Autodesk Inventor part; units mm, degrees
ref_plane "Work Plane1" through (0, 0, -15) normal (0, 0, 1) x (1, 0, 0)
ref_plane "YZ Plane" through (0, 0, 0) normal (1, 0, 0) x (0, 1, 0)
ref_plane "XZ Plane" through (0, 0, 0) normal (0, 1, 0) x (-1, 0, 0)
sketch "Sketch1" plane through (0, 0, 0) normal (0, 0, 1) x (1, 0, 0)
  line L0 (0, 0) -> (25, 0)
  line L1 (25, 0) -> (25, 40)
  line L2 (25, 40) -> (0, 40)
  line L3 (0, 40) -> (0, 0)
  dimension "d1" = 25
  dimension "d2" = 40
  dimension "d3" = 25
extrude "Extrusion1" add sketch "Sketch1" against normal blind 30
sketch "Sketch2" plane through (25, 0, 0) normal (1, 0, 0) x (0, 0, -1)
  line L0 (0, 0) -> (30, 0)
  circle A0 centre (15, 6.56) radius 2.46
extrude "Extrusion2" cut sketch "Sketch2" against normal blind 30
sketch "Sketch3" plane through (0, 0, 0) normal (-1, 0, 0) x (0, 0, 1)
  line L0 (0, 0) -> (-30, 0)
  line L1 (-25.05, 0) -> (-4.95, 0)
  line L2 (-4.95, 0) -> (-4.95, 33.12)
  line L3 (-4.95, 33.12) -> (-25.05, 33.12)
  line L4 (-25.05, 33.12) -> (-25.05, 0)
  dimension "d11" = 20.1
extrude "Extrusion3" cut sketch "Sketch3" against normal blind 20
sketch "Sketch4" plane through (0, 0, 0) normal (0, -1, 0) x (1, 0, 0)
  line L0 (20, -4.95) -> (20, -25.05)
  line L1 (20, -15) -> (25, -15)
  line L2 (25, 0) -> (25, -30)
  line L3 (20, -8.025) -> (25, -8.025)
  line L4 (25, -8.025) -> (25, -21.975)
  line L5 (25, -21.975) -> (20, -21.975)
  line L6 (20, -21.975) -> (20, -8.025)
  line L7 (20, -8.025) -> (25, -21.975) construction
  line L8 (25, -8.025) -> (20, -21.975) construction
  line L9 (25, -12.54) -> (25, -17.46)
  point P0 (0, 0)
  point P1 (22.5, -15)
  dimension "d14" = 13.95
extrude "Extrusion4" add sketch "Sketch4" along normal blind 15
sketch "Sketch5" plane through (20, 0, 0) normal (-1, 0, 0) x (0, 0, 1)
  circle A0 centre (-15, 6.56) radius 2.46
  circle A1 centre (-15, 6.56) radius 4.7025
  circle A2 centre (-15, 6.56) radius 2.46
  circle A3 centre (-15, 6.56) radius 2.46
  point P0 (0, 0)
  dimension "d17" = 9.405
extrude "Extrusion5" cut sketch "Sketch5" against normal blind 2.1
sketch "Sketch6" plane through (25, 0, 0) normal (1, 0, 0) x (0, 0, -1)
  circle A0 centre (15, 6.56) radius 4.7025
  line L0 (15, 6.56) -> (15, 23.56)
  circle A1 centre (15, 23.56) radius 2.46
  point P0 (0, 0)
  dimension "d20" = 17
  dimension "d21" = 4.92
extrude "Extrusion6" cut sketch "Sketch6" against normal blind 10 contours A1
sketch "Sketch7" plane through (20, 0, 0) normal (-1, 0, 0) x (0, 0, 1)
  circle A0 centre (-15, 23.56) radius 2.46
  circle A1 centre (-15, 23.56) radius 4.7025
  point P0 (0, 0)
  dimension "d24" = 9.405
extrude "Extrusion7" cut sketch "Sketch7" against normal blind 2.1
sketch "Sketch9" plane through (25, 0, 0) normal (1, 0, 0) x (0, 0, -1)
  circle A0 centre (15, 6.56) radius 2.46
  circle A1 centre (15, 6.56) radius 2.46
  circle A2 centre (15, 23.56) radius 2.46
  circle A3 centre (15, 23.56) radius 2.46
  line L0 (30, 40) -> (30, 0)
  line L1 (30, 0) -> (30, 40)
  line L2 (30, 40) -> (0, 40)
  line L3 (0, 40) -> (0, 0)
  line L4 (0, 0) -> (8.025, 0)
  line L5 (21.975, 0) -> (21.975, -15)
  line L6 (21.975, -15) -> (8.025, -15)
  line L7 (8.025, -15) -> (8.025, 0)
  line L8 (0, 0) -> (8.025, 0)
  line L9 (21.975, 0) -> (30, 0)
extrude "Extrusion8" add sketch "Sketch9" along normal blind 5
sketch "Sketch10" plane through (0, 40, 0) normal (0, 1, 0) x (1, 0, 0)
  line L0 (0, 30) -> (30, 30)
  line L1 (30, 0) -> (0, 0)
  line L2 (0, 30) -> (30, 30)
  line L3 (30, 30) -> (30, 0)
  line L4 (30, 0) -> (0, 0)
  line L5 (0, 0) -> (0, 30)
extrude "Extrusion9" add sketch "Sketch10" along normal blind 30
sketch "Sketch12" plane through (30, 0, 0) normal (1, 0, 0) x (0, 0, -1)
  circle A0 centre (15, 6.56) radius 2.46
  line L0 (15, 6.56) -> (15, 15.06)
  circle A1 centre (15, 15.06) radius 2.525
  point P0 (0, 0)
  dimension "d31" = 8.5
  dimension "d33" = 5.05
extrude "Extrusion10" cut sketch "Sketch12" against normal blind 30 contours A1
sketch "Sketch14" plane through (0, 0, 0) normal (0, 0, 1) x (1, 0, 0)
  line L0 (30, 70) -> (0, 70)
  line L1 (0, 70) -> (0, 85)
  line L2 (30, 100) -> (15, 115)
  line L3 (-12, 115) -> (15, 115)
  line L4 (30, 0) -> (30, 70)
  line L5 (30, 100) -> (30, 70)
  line L6 (-9.5, 113.5) -> (-12, 115)
  line L7 (-9.5, 101.5) -> (-12, 100)
  line L8 (-7, 107.5) -> (-9.5, 101.5)
  line L9 (-7, 107.5) -> (-9.5, 113.5)
  line L10 (0, 100) -> (0, 85)
  line L11 (0, 100) -> (-12, 100)
  point P0 (0, 0)
  dimension "d49" = 15
  dimension "d61" = 12
extrude "Extrusion12" add sketch "Sketch14" against normal blind 30
sketch "Sketch15" plane through (0, 0, -25.05) normal (-1, 0, 0) x (0, 0, 1)
  line L0 (0, 33.12) -> (20.1, 33.12)
  line L1 (20.1, 33.12) -> (20.1, 0)
  line L2 (0, 33.12) -> (20.1, 33.12)
  line L3 (20.1, 33.12) -> (20.1, 31.1)
  line L4 (20.1, 31.1) -> (0, 31.1)
  line L5 (0, 31.1) -> (0, 33.12)
  point P0 (25.05, 0)
  dimension "d57" = 2.02
extrude "Extrusion13" add sketch "Sketch15" against normal blind 20
sketch "Sketch19" plane through (0, 0, 0) normal (0, 0, 1) x (1, 0, 0)
  line L0 (0, 100) -> (0, 0)
  line L1 (0, 100) -> (-12, 100)
  line L2 (0, 100) -> (-12, 100)
  line L3 (-12, 100) -> (-9.5, 101.5)
  line L4 (-12, 100) -> (-9.5, 101.5)
  line L5 (-9.5, 101.5) -> (-7, 107.5)
  line L6 (-9.5, 101.5) -> (-7, 107.5)
  line L7 (-7, 107.5) -> (-9.5, 113.5)
  line L8 (-7, 107.5) -> (-9.5, 113.5)
  line L9 (-9.5, 113.5) -> (-12, 115)
  line L10 (-9.5, 113.5) -> (-12, 115)
  line L11 (-12, 115) -> (15, 115)
  line L12 (-12, 115) -> (15, 115)
  line L13 (15, 115) -> (30, 100)
  line L14 (15, 115) -> (30, 100)
  line L15 (30, 100) -> (30, 90)
  line L16 (30, 0) -> (30, 100)
  line L17 (30, 90) -> (0, 90)
  line L18 (0, 0) -> (0, 100)
  line L19 (0, 90) -> (0, 100)
  dimension "d62" = 10
  dimension "d63" = 30
extrude "Extrusion14" add sketch "Sketch19" along normal blind 15
ref_plane "Work Plane1" through (0, 0, -15) normal (0, 0, 1) x (1, 0, 0)
mirror "Mirror1" about plane through (0, 0, -15) normal (0, 0, 1) of "Extrusion14"
properties part number "rec_b_12mm_x_60mm"
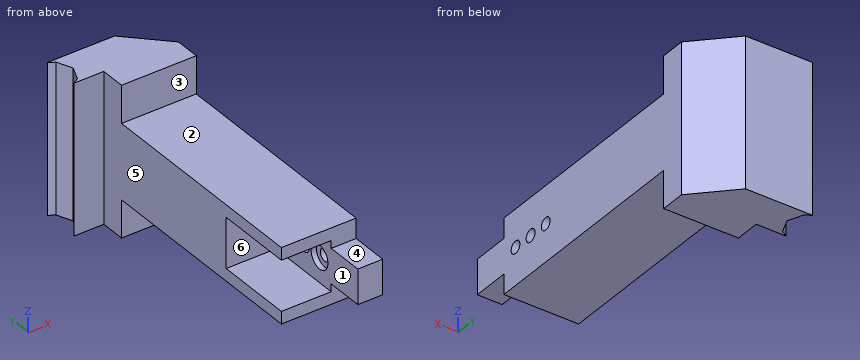
Build history of the part. All positions in model axes, mm. Face numbers are marked on the shaded views. A direction names the side the tool comes from. Round coordinates to 2 decimals unless told otherwise and drop trailing zeros. Write each loop counter-clockwise with the first axis right and the second up, starting at its lowest first coordinate (ties: lowest second). Pieces come first, ordered by that corner, then holes.
1) Band-saw the part on B-B, the plane z = -15. Give the number of separate pieces and of enclosed holes in the cut face, and give its area (3 significant figures).
2) Band-saw the part on A-A, the plane y = 15.06. List the corners of the cut face in (x, z) (3 decimals), and give its area (4 significant figures).
3) Pin check, flat tips, straight feed: pin 1 (2.5 mm diameter, centred on x = 15.5, z = -2.5, fed in from -Y); pin 2 (10 mm diameter, centred on y = -2.5, z = -16, fed in from -X); pin 3 (24 mm diameter, centred on x = 11.5, y = 44, fed in from +Z); pin 4 (4 mm diameter, centred on y = 23.56, z = -15, fed in from -X). Stop position of each tip, or through.
4) Band-saw the part on C-C, the plane x = 18.5. List the corners of the cut face in (y, z).
5) Drill centre lines: probe 1 along Z at (x, y) = (9.5, 19.5); probe 2 along Y at (x, z) = (26, -15) (3 decimals); probe 3 along Z at (x, y) = (26.25, 23.56). Where is each one in solid material? Low to high.
6) 3-axis set-ups, long thin cutter, end or side, ignore diameter. For the marked faces 4, 5 and 6: which of +Z, -Z, +X, -X, +Y, -Y reach the whole face in a straight line?
7) Mould opens along Z. For the marked faces 1, 2 and 3 say: +Z half, -Z half, draft (parallel to the pull), parting line (faces both ways), or undercut.
8) Band-saw the part on D-D, the plane y = 97.5. List the corners of the cut face in (x, z), and give its area (3 significant figures).
Ans:
1. separate pieces: 4
1. enclosed holes: 0
1. area: 2,830 mm2
2. outline: (0, -30) - (30, -30) - (30, -17.525) - (20, -17.525) - (20, -25.05) - (0, -25.05) - close; (0, -4.95) - (20, -4.95) - (20, -12.475) - (30, -12.475) - (30, 0) - (0, 0) - close
2. area: 447.5 mm2
3. pin 1: stops at y = 0
3. pin 2: stops at x = 20
3. pin 3: stops at z = 0
3. pin 4: passes through
4. outline: (0, -30) - (90, -30) - (90, -45) - (111.5, -45) - (111.5, 15) - (90, 15) - (90, 0) - (0, 0) - (0, -4.95) - (31.1, -4.95) - (31.1, -25.05) - (0, -25.05) - close
5. probe 1: z = -30 to -25.05, -4.95 to 0
5. probe 2: y = -15 to 4.1, 9.02 to 12.535, 17.585 to 21.1, 26.02 to 104
5. probe 3: z = -30 to -17.46, -12.54 to 0
6. face 4: +Z, +X, -X, -Y
6. face 5: +Z, -Z, -X, -Y
6. face 6: -X, -Y
7. face 1: undercut
7. face 2: +Z half
7. face 3: draft
8. outline: (0, -45) - (30, -45) - (30, 15) - (0, 15) - close
8. area: 1,800 mm2
